The listing builds one solid part. Answer for the finished solid, in the listing's coordinates (mm). A direction names the side the tool comes from. Coordinates: 2 decimals unless noted, no trailing zeros. Order: outer loops, then holes, each group sorted by start corner. A loop starts at its lowest first (then second) coordinate and runs counter-clockwise, first axis right, second up.
```python
from build123d import *

# Parameters (mm, degrees)
BOSS_EXTRUDE1_DEPTH = 3
SKETCH4_W           = 30
SKETCH4_H           = 46
CUT_EXTRUDE1_DEPTH  = 3
FILLET1_R           = 5
FILLET2_R           = 1
SKETCH5_R           = 1.5
SKETCH5_R_2         = 2
CUT_EXTRUDE2_DEPTH  = 3


with BuildPart() as part:
    # Sketch1 → Boss-Extrude1 (new body)
    with BuildSketch(Plane(origin=(0, 0, 0), x_dir=(1, 0, 0), z_dir=(0, 1, 0))):
        Polygon((0, -32.526631134), (27.473368866, -60), (190, -60), (190, 60), (27.473368866, 60), (0, 32.526631134), (0, 23), (0, -23), align=None)
    extrude(amount=BOSS_EXTRUDE1_DEPTH)

    # Sketch4 → Cut-Extrude1 (cut)
    with BuildSketch(Plane(origin=(0, 0, 0), x_dir=(1, 0, 0), z_dir=(0, 1, 0))):
        Polygon((68.526631134, -60), (68.526631134, -52.5), (62.526631134, -52.5), (62.526631134, -40.526631134), (55, -33), (35, -33), (27.473368866, -40.526631134), (27.473368866, -52.5), (19.973368866, -52.5), (27.473368866, -60), align=None)
        Polygon((27.473368866, 60), (68.526631134, 60), (68.526631134, 52.5), (62.526631134, 52.5), (62.526631134, 40.526631134), (55, 33), (35, 33), (27.473368866, 40.526631134), (27.473368866, 52.5), (19.973368866, 52.5), align=None)
        with Locations((15, 0)):
            Rectangle(SKETCH4_W, SKETCH4_H)
    extrude(amount=CUT_EXTRUDE1_DEPTH, mode=Mode.SUBTRACT)

    # Fillet1
    fillet1_edges = [part.edges().sort_by_distance(p)[0] for p in [
        (190, 1.5, -60),
        (190, 1.5, 60),
        (0, 1.5, 32.526631134),
        (0, 1.5, -32.526631134),
        (68.526631134, 1.5, 60),
        (19.973368866, 1.5, 52.5),
        (19.973368866, 1.5, -52.5),
        (68.526631134, 1.5, -60),
    ]]
    fillet(fillet1_edges, radius=FILLET1_R)

    # Fillet2
    fillet2_edges = [part.edges().sort_by_distance(p)[0] for p in [
        (68.526631134, 1.5, 52.5),
        (68.526631134, 1.5, -52.5),
    ]]
    fillet(fillet2_edges, radius=FILLET2_R)

    # Sketch5 → Cut-Extrude2 (cut)
    with BuildSketch(Plane(origin=(0, 0, 0), x_dir=(1, 0, 0), z_dir=(0, 1, 0))):
        with Locations((47.062554885, -18.5)):
            Circle(SKETCH5_R)
        with Locations((84.062554885, -18.5)):
            Circle(SKETCH5_R)
        with Locations((84.062554885, 18.5)):
            Circle(SKETCH5_R)
        with Locations((47.062554885, 18.5)):
            Circle(SKETCH5_R)
        with Locations((94, 23.219474586)):
            Circle(SKETCH5_R)
        with Locations((93.305417602, 33.219474586)):
            Circle(SKETCH5_R)
        with Locations((29.11536409, 34.641995223)):
            Circle(SKETCH5_R)
        with Locations((60.88463591, 34.641995223)):
            Circle(SKETCH5_R)
        with Locations((8.367356219, -27.085410895)):
            Circle(SKETCH5_R)
        with Locations((16.379446424, 26.606355181)):
            Circle(SKETCH5_R)
        with Locations((94, -30.308001182)):
            Circle(SKETCH5_R)
        with Locations((86.659783805, -40.308001182)):
            Circle(SKETCH5_R)
        with Locations((184, -45)):
            Circle(SKETCH5_R)
        with Locations((184, 45)):
            Circle(SKETCH5_R)
        with Locations((166, -19.5)):
            Circle(SKETCH5_R_2)
        with Locations((166, 19.5)):
            Circle(SKETCH5_R_2)
        with Locations((29.11536409, -34.641995223)):
            Circle(SKETCH5_R)
        with Locations((60.88463591, -34.641995223)):
            Circle(SKETCH5_R)
        with Locations((21.933678109, -25.25)):
            Circle(SKETCH5_R)
        with Locations((5.439723212, 25.25)):
            Circle(SKETCH5_R)
    extrude(amount=CUT_EXTRUDE2_DEPTH, mode=Mode.SUBTRACT)


solid = part.part
```
1) For faces 4 (the flat face through (9.867, 1.479, 42.394)), 5 (the flat face through (59, 1, -37)), 6 (the flat face through (59, 1, 37)), determine the directions among +Z, -Z, +X, -X, +Y, -Y from which every point of the face is accessible in a straight line to the end or side of a thin tool.
2) Straight lines are drawn through the part: probe 1 along Z at (x, y) = (166, 0.9); probe 2 along X at (y, z) = (0.7, 45); probe 3 along Z at (x, y) = (8, 1.5). For each, find the intervals that lie inside material, in ascending order.
3) The mould has two halves that part along X. Classify faces 1 (the cylindrical face through (189, 2, 58)), 2 (the cylindrical face through (164.002, 1.479, 19.412)), 3 (the flat face through (115, 0, -1)): released by +X, released by -X, zero draft, split by the parting line, or undercut.
4) A cutting plane is placed at C-C, the plane x = 39.5. Write down the section's boundary in (y, z).
5) Each of these flat-tipped pins is pushed along its axis until it touches: P1, Ø1.8, axis at x = 60.88, z = 34.64, coming from the +Y side; P2, Ø1.5, axis at x = 62.5, y = 2.5, coming from the +Z side; P3, Ø1.6, axis at y = 2, z = -54, coming from the -X side; P4, Ø1.5, axis at x = 15, y = 2, coming from the -Z side. Where does it stop, or does it pass through?
6) A cutting plane is placed at A-A, the plane x = 166. Write down the section's boundary in (y, z).
7) A cutting plane is placed at B-B, the plane z = 7. Write down the section's boundary in (x, y).
8) A cutting plane is placed at D-D, the plane y = 1.4. Count the separate pieces of the cut face and the enclosed holes in it, plus the area to 3 significant figures.
Working result:
1. face 4: +Z, -X, +Y, -Y
1. face 5: -Z, +Y, -Y
1. face 6: +Z, +Y, -Y
2. probe 1: z = -60 to -21.5, -17.5 to 17.5, 21.5 to 60
2. probe 2: x = 12.47 to 27.47, 62.53 to 182.5, 185.5 to 190
2. probe 3: z = -40.53 to -23, 23 to 25.63, 28.54 to 40.53
3. face 1: released by +X
3. face 2: undercut
3. face 3: zero draft
4. outline: (0, -33) - (3, -33) - (3, 33) - (0, 33) - close
5. P1: passes through
5. P2: stops at z = 52.5
5. P3: stops at x = 68.48
5. P4: stops at z = -48.28
6. outline: (0, -60) - (3, -60) - (3, -21.5) - (0, -21.5) - close; (0, -17.5) - (3, -17.5) - (3, 17.5) - (0, 17.5) - close; (0, 21.5) - (3, 21.5) - (3, 60) - (0, 60) - close
7. outline: (30, 0) - (190, 0) - (190, 3) - (30, 3) - close
8. separate pieces: 1
8. enclosed holes: 20
8. area: 18,600 mm2
